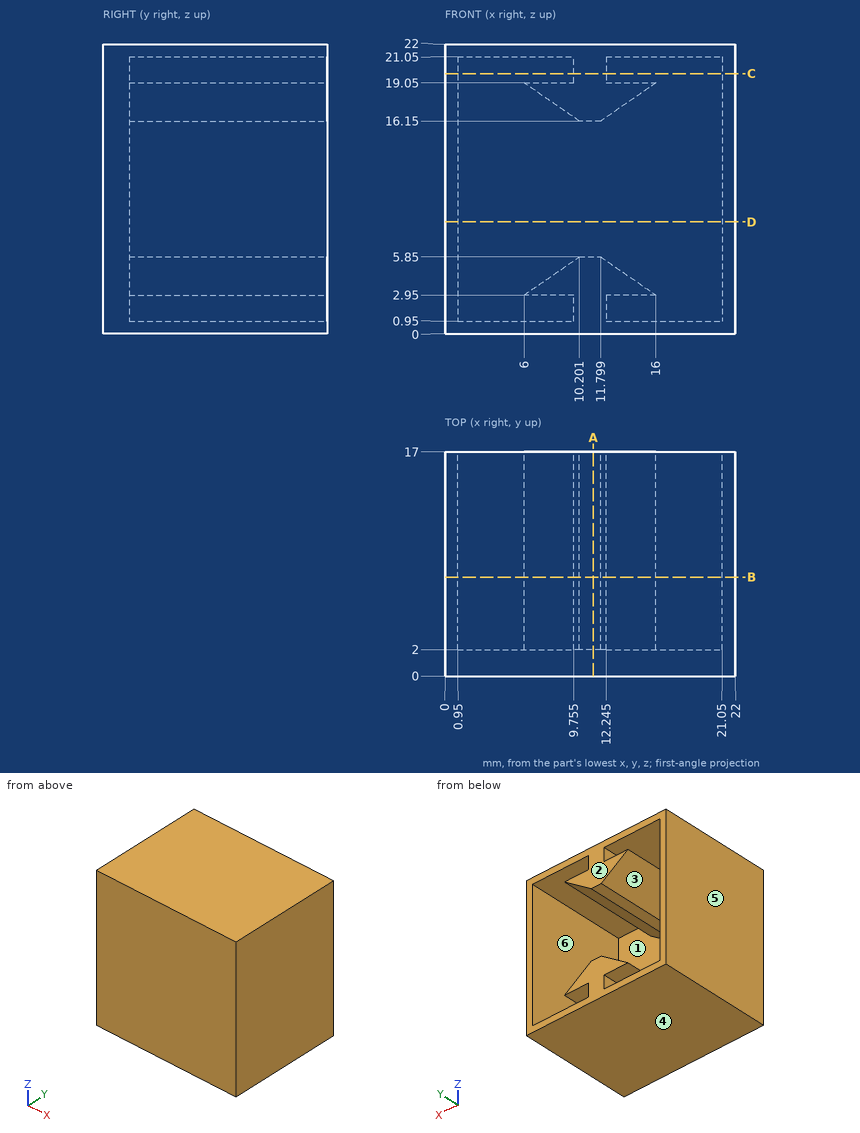
Geometry check sheet. Reference: drawing and pictorial views, mm from the part's lowest x, y, z. A direction names the side the tool comes from. Coordinates: 2 decimals unless noted, no trailing zeros. Write each loop counter-clockwise with the first axis right and the second up, starting at its lowest first coordinate (ties: lowest second). Pieces come first, ordered by that corner, then holes. Notation, with made-up numbers: M -26,26 L 1,26 A25 cw 1,59 Z; hole C 47,26.5 d3. An arc over 180 degrees is marked long. Write item = value, one per line. Start each with the question number.
1. Sectioned sample at B-B (y = 7.5). Record the cut outline in (x, z) (3 decimals).
2. Thickness scan on probe 1 along X at (y, z) = (4, 19.5) (3 decimals); probe 2 along Z at (x, y) = (18.25, 7.75); probe 3 along Z at (x, y) = (13, 2.25). Record the ranges inside material, lowest first.
3. Sectioned sample at D-D (z = 8.5). Record the cut outline in (x, y).
4. Sectioned sample at A-A (x = 11.25). Record the cut outline in (y, z).
5. Tool access check on the marked faces 5 and 6. Record the directions out of +Z, -Z, +X, -X, +Y, -Y that give a thin tool (end or side, any length) a straight path to the whole face; none if there is none.
6. Mould release check, pull along Z, two halves, no side actions. Record for the marked faces 1, 2, 3 and 4: pulls with the +Z half, pulls with the -Z half, needs draft (parallel to the pull), parting line crosses it, or undercut.
7. Sectioned sample at C-C (z = 19.75). Record the cut outline in (x, y) (3 decimals).
8. Go/stop test with a flat-tipped pin: pin 1 (6 mm diameter, centred on x = 9, z = 12.5, fed in from +Y). Record where the tip stops, or that it passes through.
The answers:
q1.outline = M 0,0 L 22,0 L 22,22 L 0,22 Z; hole M 0.95,0.95 L 9.755,0.95 L 9.755,2.95 L 6,2.95 L 10.201,5.85 L 11.799,5.85 L 16,2.95 L 12.245,2.95 L 12.245,0.95 L 21.05,0.95 L 21.05,21.05 L 12.245,21.05 L 12.245,19.05 L 16,19.05 L 11.799,16.15 L 10.201,16.15 L 6,19.05 L 9.755,19.05 L 9.755,21.05 L 0.95,21.05 Z
q2.probe_1 = 0 to 0.95, 9.755 to 12.245, 21.05 to 22
q2.probe_2 = 0 to 0.95, 21.05 to 22
q2.probe_3 = 0 to 0.95, 2.95 to 5.02, 16.98 to 19.05, 21.05 to 22
q3.outline = M 0,0 L 22,0 L 22,17 L 21.05,17 L 21.05,2 L 0.95,2 L 0.95,17 L 0,17 Z
q4.outline = M 0,0 L 17,0 L 17,5.85 L 2,5.85 L 2,16.15 L 17,16.15 L 17,22 L 0,22 Z
q5.face_5 = +Z, -Z, -X, +Y, -Y
q5.face_6 = +Y
q6.face_1 = undercut
q6.face_2 = needs draft
q6.face_3 = undercut
q6.face_4 = pulls with the -Z half
q7.outline = M 0,0 L 22,0 L 22,17 L 21.05,17 L 21.05,2 L 12.245,2 L 12.245,17 L 9.755,17 L 9.755,2 L 0.95,2 L 0.95,17 L 0,17 Z
q8.pin_1 = 2
